Verification items for this drawing (mm, ordinates from the low corner). Give positions to 0.01 mm unless a question says otherwise; leave off trailing zeros. Loops run counter-clockwise (first coordinate to the right, second up) from the corner with the lowest first, then second, coordinate; pieces in that order, holes last. Notation, with made-up numbers: (55.25, -23) -> (63.25, -23) arc R28 cw to (63.25, -4) -> close; hole circle Ø10 at (48.25, -33). An arc over 180 degrees is marked (long way). Write each question's results on one line, items separated by ' | '. Start each with the question number.
Item 1: Gauge pin test, flat ends, axial feed: pin 1 Ø6 at (x, z) = (92.5, 26.5) entering from -Y; pin 2 Ø1 at (x, y) = (17, 2) entering from +Z. Record the tip position at first contact, or that the pin passes through.
Item 2: Cross-section at C-C on x = 52. Enter the section's corners in (y, z) (1 decimal).
Item 3: Mould release check, pull along Y, two halves, no side actions. Record for the marked faces 1 and 2: pulls with the +Y half, pulls with the -Y half, needs draft (parallel to the pull), parting line crosses it, or undercut.
Item 4: Cross-section at B-B on z = 102.5. Enter the section's corners in (x, y).
Item 5: Scan lines: line 1 along Z through (x, y) = (116, 1.4); line 2 along Z through (x, y) = (40, 0.85); line 3 along X through (y, z) = (2.2, 42). Record each from-to range of solid material in increasing order.
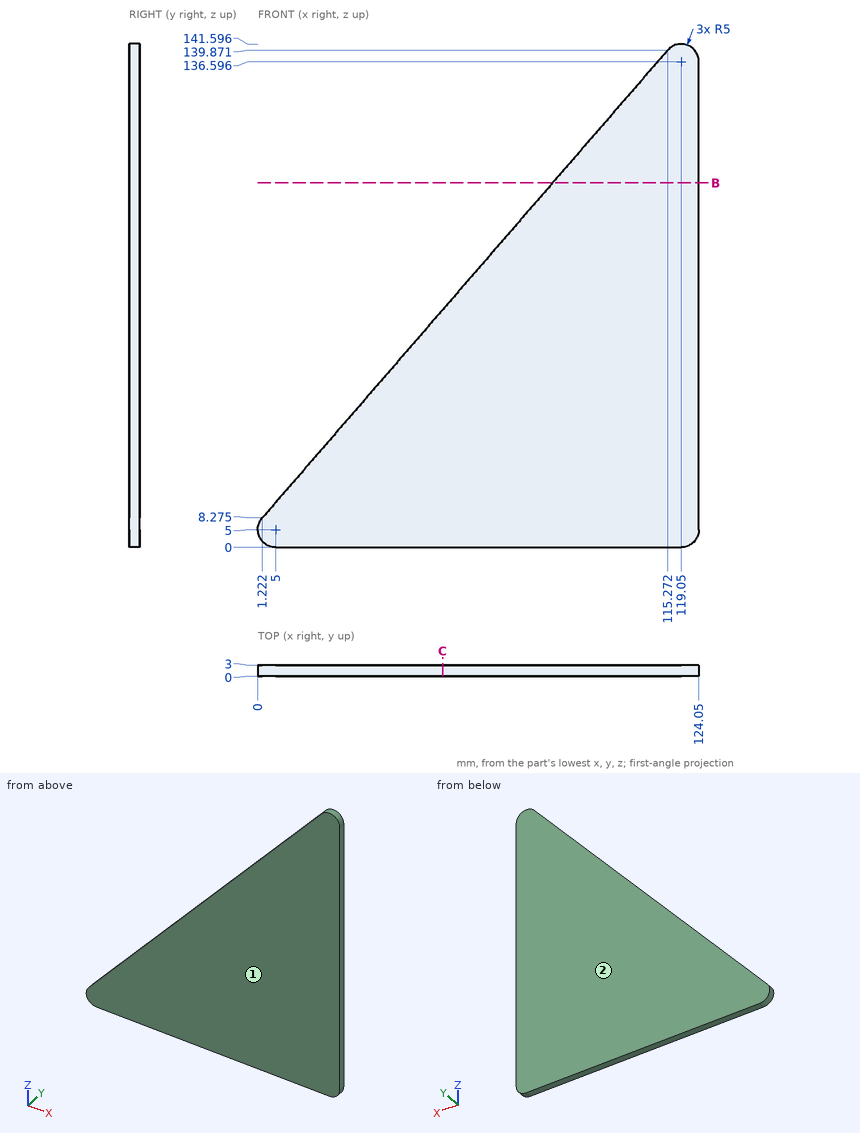
Answer sheet:
1) pin 1: stops at y = 0 | pin 2: stops at z = 27.06
2) outline: (0, 0) -> (3, 0) -> (3, 66.9) -> (0, 66.9) -> close
3) face 1: pulls with the -Y half | face 2: pulls with the +Y half
4) outline: (82.88, 0) -> (124.05, 0) -> (124.05, 3) -> (82.88, 3) -> close
5) line 1: z = 0 to 140.56 | line 2: z = 0 to 53.02 | line 3: x = 30.45 to 124.05
